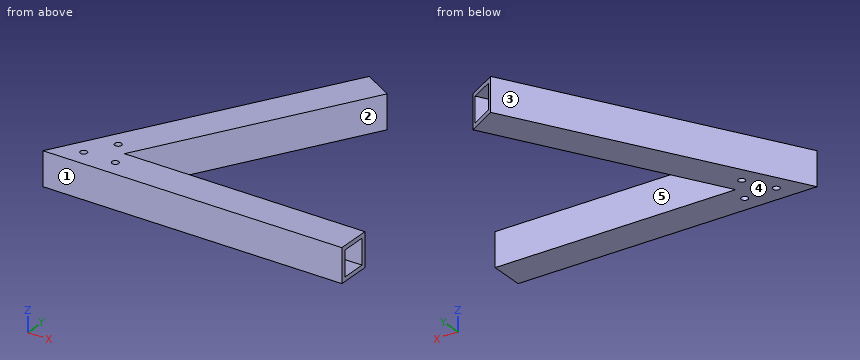
Autodesk Inventor part; units mm, degrees
ref_plane "YZ Plane" through (0, 0, 0) normal (1, 0, 0) x (0, 1, 0)
ref_plane "XZ Plane" through (0, 0, 0) normal (0, 1, 0) x (-1, 0, 0)
ref_plane "XY Plane" through (0, 0, 0) normal (0, 0, 1) x (1, 0, 0)
sketch "Sketch1" plane through (0, 0, 0) normal (0, 0, 1) x (1, 0, 0)
  line L0 (0, 0) -> (-203.2, 0)
  line L1 (-203.2, 0) -> (-101.6, 175.9764)
  dimension "d0" = 60
  dimension "d1" = 203.2
sketch "Sketch2" plane through (0, 0, 0) normal (1, 0, 0) x (0, 1, 0)
  line L0 (-12.7, 12.7) -> (-12.7, -12.7)
  line L1 (-12.7, -12.7) -> (12.7, -12.7)
  line L2 (12.7, -12.7) -> (12.7, 12.7)
  line L3 (12.7, 12.7) -> (-12.7, 12.7)
  line L4 (-12.7, 12.7) -> (12.7, -12.7) construction
  line L5 (-12.7, -12.7) -> (12.7, 12.7) construction
  line L6 (-9.525, 9.525) -> (-9.525, -9.525)
  line L7 (-9.525, -9.525) -> (9.525, -9.525)
  line L8 (9.525, -9.525) -> (9.525, 9.525)
  line L9 (9.525, 9.525) -> (-9.525, 9.525)
  line L10 (-9.525, 9.525) -> (9.525, -9.525) construction
  line L11 (-9.525, -9.525) -> (9.525, 9.525) construction
  point P0 (0, 0)
  dimension "d2" = 25.4
  dimension "d3" = 3.175
sweep "Sweep1" add profiles "Sketch2" path "Sketch1"
sketch "Sketch3" plane through (0, -12.7, 12.7) normal (0, 0, 1) x (1, 0, 0)
  line L0 (0, 0) -> (-225.197, 0) construction
  line L1 (0, 25.4) -> (-181.203, 25.4) construction
  line L2 (-225.197, 0) -> (-181.203, 25.4) construction
  circle A0 centre (-203.2, 12.7) radius 2.54
  line L3 (-112.5985, 195.0264) -> (-90.6015, 182.3264) construction
  line L4 (-190.0237, 35.5219) -> (-203.2, 12.7) construction
  line L5 (-203.2, 12.7) -> (-176.8475, 12.7) construction
  circle A1 centre (-191.2937, 33.3222) radius 2.54
  circle A2 centre (-179.3875, 12.7) radius 2.54
  point P0 (0, 12.7)
  dimension "d6" = 5.08
  dimension "d10" = 23.8125
extrude "Extrusion1" cut sketch "Sketch3" against normal through all
properties part number "60DegreeAlumTubing"
Work out the finished part from the listing and answer in its coordinate system (mm). Face numbers are marked on the shaded views. A direction names the side the tool comes from. Coordinates: 2 decimals unless noted, no trailing zeros. Loops run counter-clockwise (first coordinate to the right, second up) from the corner with the lowest first, then second, coordinate; pieces in that order, holes last. Notation, with made-up numbers: (63.5, -31) - (77.5, -31) arc R26 ccw to (77.5, -2) - close; hole circle Ø9 at (41, 36). An arc over 180 degrees is marked (long way). Use a Markdown table: item, result.
Item 1: Given pin 1 Ø12 at (y, z) = (130.5, -10) entering from +X; pin 2 Ø6 at (y, z) = (75, 8.5) entering from -X; pin 3 Ø12 at (y, z) = (98.5, -4) entering from -X, each flat-ended and moving along its own axis, determine where each tip first touches the part or whether it passes through.
Evaluation:
| item | result |
|---|---|
| pin 1 | stops at x = -109.73 |
| pin 2 | stops at x = -176.3 |
| pin 3 | stops at x = -164.46 |
Item 2: Find section D-D, the plane y = 0. Determine the outline of the cut face in (x, z) (1 decimal).
Evaluation:
| item | result |
|---|---|
| outline | (-217.9, -12.7) - (-205.7, -12.7) - (-205.7, -9.5) - (-214.2, -9.5) - (-214.2, 9.5) - (-205.7, 9.5) - (-205.7, 12.7) - (-217.9, 12.7) - close; (-200.7, -12.7) - (-181.9, -12.7) - (-181.9, -9.5) - (-200.7, -9.5) - close; (-200.7, 9.5) - (-181.9, 9.5) - (-181.9, 12.7) - (-200.7, 12.7) - close; (-176.8, -12.7) - (0, -12.7) - (0, -9.5) - (-176.8, -9.5) - close; (-176.8, 9.5) - (0, 9.5) - (0, 12.7) - (-176.8, 12.7) - close |
Item 3: Consider probe 1 along Y at (x, z) = (-178.5, -2.5) (3 decimals); probe 2 along Y at (x, z) = (-123, -3) (1 decimal); probe 3 along Z at (x, y) = (-113.5, 141) (3 decimals). Determine where each line is inside the solid, lowest interval first. Write a range as from..to.
Evaluation:
| item | result |
|---|---|
| probe 1 | y = -12.7..-9.525, 9.525..12.7, 17.382..23.732, 61.832..68.182 |
| probe 2 | y = -12.7..-9.5, 9.5..12.7, 113.5..119.9, 158..164.3 |
| probe 3 | z = -12.7..-9.525, 9.525..12.7 |
Item 4: Find section B-B, the plane x = -203.2. Determine the outline of the cut face in (y, z) (3 decimals).
Evaluation:
| item | result |
|---|---|
| outline | (-12.7, -12.7) - (-2.54, -12.7) - (-2.54, -9.525) - (-9.525, -9.525) - (-9.525, 9.525) - (-2.54, 9.525) - (-2.54, 12.7) - (-12.7, 12.7) - close; (2.54, -12.7) - (25.4, -12.7) - (25.4, 12.7) - (2.54, 12.7) - (2.54, 9.525) - (19.05, 9.525) - (19.05, -9.525) - (2.54, -9.525) - close |
Item 5: Find section A-A, the plane x = -85.5. Determine the outline of the cut face in (y, z) (3 decimals).
Evaluation:
| item | result |
|---|---|
| outline | (-12.7, -12.7) - (12.7, -12.7) - (12.7, 12.7) - (-12.7, 12.7) - close; hole (-9.525, -9.525) - (9.525, -9.525) - (9.525, 9.525) - (-9.525, 9.525) - close |
Item 6: The mould has two halves that part along Y. Classify the marked faces 3, 4 and 5: +Y half, -Y half, draft (parallel to the pull), parting line (faces both ways), or undercut.
Evaluation:
| item | result |
|---|---|
| face 3 | +Y half |
| face 4 | draft |
| face 5 | undercut |
Item 7: For the marked faces 1 and 2, determine the directions among +Z, -Z, +X, -X, +Y, -Y from which every point of the face is accessible in a straight line to the end or side of a thin tool.
Evaluation:
| item | result |
|---|---|
| face 1 | +Z, -Z, +X, -X, -Y |
| face 2 | +Z, -Z, +X |
Item 8: Find section C-C, the plane z = -7. Determine the outline of the cut face in (x, y) (3 decimals).
Evaluation:
| item | result |
|---|---|
| outline | (-225.197, -12.7) - (0, -12.7) - (0, -9.525) - (-219.698, -9.525) - (-109.849, 180.739) - (-112.599, 182.326) - close; (-186.702, 9.525) - (0, 9.525) - (0, 12.7) - (-181.203, 12.7) - (-90.601, 169.626) - (-93.351, 171.214) - close |
